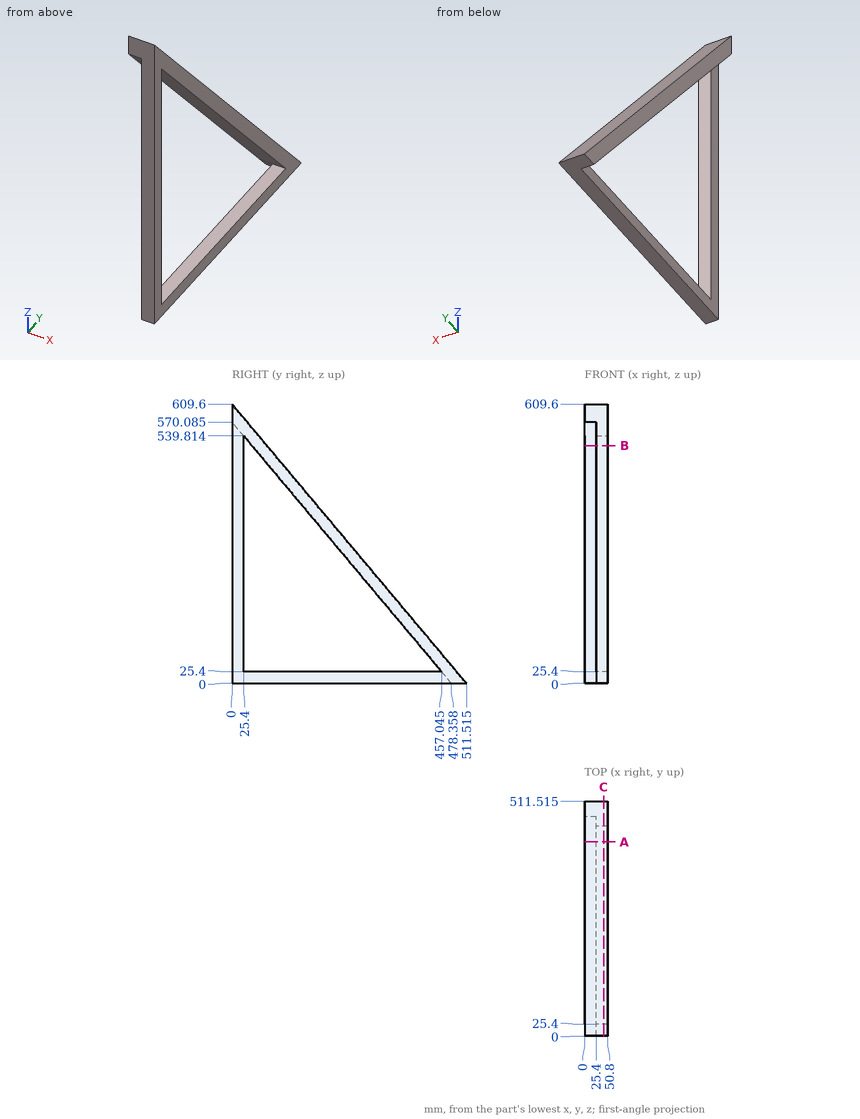
For this review, use the dimensioned drawing (mm, ordinates from the lowest corner) and the shaded views. Coordinates: 2 decimals unless noted, no trailing zeros. Loops run counter-clockwise (first coordinate to the right, second up) from the corner with the lowest first, then second, coordinate; pieces in that order, holes last. Notation, with made-up numbers: (-6, 51.25) -> (38, 51.25) arc R23 cw to (38, 65.25) -> close; hole circle Ø4 at (55, 38). An arc over 180 degrees is marked (long way). Use a Markdown table: item, result. Add a question column.
Item 1: We need section C-C, the plane x = 41.5. Write out the cut boundary in (y, z) (1 decimal), and give its area (3 significant figures).
Item 2: Clearance check with flat-ended pins moving along their axes: P1, Ø7.5, axis at x = 37, y = 331.5, coming from the +Z side; P2, Ø2, axis at x = 33.5, y = 365.5, coming from the +Z side (1 decimal); P3, Ø1, axis at x = 23, y = 331.5, coming from the -Z side. State where each tip first meets the part, or that it passes through.
Item 3: Wall thickness on L1, parallel to Z at x = 26, y = 147.5 (1 decimal); L2, parallel to Z at x = 47, y = 288 (1 decimal); L3, parallel to Y at x = 32, z = 73 (1 decimal): over which ranges is each line inside the solid? List them lowest first. Write a range as from..to.
Item 4: We need section A-A, the plane y = 423.5. Write out the cut boundary in (x, z).
Item 5: We need section B-B, the plane z = 519. Write out the cut boundary in (x, y) (1 decimal).
Numbers:
| question | item | result |
|---|---|---|
| 1 | outline | (0, 0) -> (511.5, 0) -> (0, 609.6) -> close; hole (25.4, 25.4) -> (457, 25.4) -> (25.4, 539.8) -> close |
| 1 | area | 44,900 mm^2 |
| 2 | P1 | stops at z = 219 |
| 2 | P2 | stops at z = 175.2 |
| 2 | P3 | stops at z = 174.42 |
| 3 | L1 | z = 0..25.4, 394.3..433.8 |
| 3 | L2 | z = 0..25.4, 226.9..266.4 |
| 3 | L3 | y = 0..25.4, 417.1..450.3 |
| 4 | outline | (0, 65.38) -> (50.8, 65.38) -> (50.8, 104.89) -> (0, 104.89) -> close; (25.4, 0) -> (50.8, 0) -> (50.8, 25.4) -> (25.4, 25.4) -> close |
| 5 | outline | (0, 42.9) -> (50.8, 42.9) -> (50.8, 76) -> (0, 76) -> close; (25.4, 0) -> (50.8, 0) -> (50.8, 25.4) -> (25.4, 25.4) -> close |
